from build123d import *

# Parameters (mm, degrees)
EXTRUDE_1_DEPTH     = 0.775
SKETCH_2_R          = 1.155
EXTRUDE_2_DEPTH     = 4.215
EXTRUDE_3_DEPTH     = 7.76
EXTRUDE_4_DEPTH     = 4.55
CUT_EXTRUDE_1_DEPTH = 2.5


with BuildPart() as part:
    # 스케치1 → 보스-돌출1 (new body, symmetric)
    with BuildSketch(Plane(origin=(0, 0, 0), x_dir=(0, 0, -1), z_dir=(1, 0, 0))):
        with BuildLine():
            Line((-2.73, 2.732106893), (-2.73, 2.198209499))
            ThreePointArc((-2.73, 2.198209499), (0, -3.505), (2.73, 2.198209499))
            Line((2.73, 2.198209499), (2.73, 2.732106893))
            ThreePointArc((2.73, 2.732106893), (0, 3.595), (-2.73, 2.732106893))
        make_face()
    extrude(amount=EXTRUDE_1_DEPTH, both=True)

    # 스케치2 → 보스-돌출2 (add, symmetric)
    with BuildSketch(Plane(origin=(0, 0, 0), x_dir=(0, 0, -1), z_dir=(1, 0, 0))):
        Circle(SKETCH_2_R)
    extrude(amount=EXTRUDE_2_DEPTH, both=True)

    # 스케치3 → 보스-돌출3 (add, symmetric)
    with BuildSketch(Plane(origin=(0, 0, 0), x_dir=(0, 0, -1), z_dir=(1, 0, 0))):
        with BuildLine():
            Line((-4.05, 2.73), (-2.73, 2.73))
            Line((-2.73, 2.73), (-2.73, 2.732106893))
            ThreePointArc((-2.73, 2.732106893), (0, 3.595), (2.73, 2.732106893))
            Line((2.73, 2.732106893), (2.73, 2.73))
            Line((2.73, 2.73), (4.05, 2.73))
            Line((4.05, 2.73), (4.05, 4.86))
            Line((4.05, 4.86), (-4.05, 4.86))
            Line((-4.05, 4.86), (-4.05, 2.73))
        make_face()
    extrude(amount=EXTRUDE_3_DEPTH, both=True)

    # 스케치4 → 보스-돌출4 (add)
    with BuildSketch(Plane(origin=(0, 4.86, 0), x_dir=(1, 0, 0), z_dir=(0, 1, 0))):
        with BuildLine():
            Line((-2.555, -2.44), (-5.335, -2.44))
            ThreePointArc((-5.335, -2.44), (-5.567190107, -1.747089472), (-6.17, -1.333982369))
            Line((-6.17, -1.333982369), (-6.17, 1.333982369))
            ThreePointArc((-6.17, 1.333982369), (-5.567190107, 1.747089472), (-5.335, 2.44))
            Line((-5.335, 2.44), (-2.555, 2.44))
            ThreePointArc((-2.555, 2.44), (-2.322809893, 1.747089472), (-1.72, 1.333982369))
            Line((-1.72, 1.333982369), (-1.72, -1.333982369))
            ThreePointArc((-1.72, -1.333982369), (-2.322809893, -1.747089472), (-2.555, -2.44))
        make_face()
    extrude_4 = extrude(amount=EXTRUDE_4_DEPTH)

    # 스케치5 → 컷-돌출1 (cut, symmetric)
    with BuildSketch(Plane.XY):
        Polygon((-6.17, 6.54), (-5.611088771, 9.41), (-6.17, 9.41), align=None)
    cut_extrude_1 = extrude(amount=CUT_EXTRUDE_1_DEPTH, both=True, mode=Mode.SUBTRACT)

    # 대칭 복사1: 보스-돌출4, 컷-돌출1 across plane
    add(extrude_4.mirror(Plane(origin=(0, 0, 0), x_dir=(0, 0, 1), z_dir=(1, 0, 0))))
    add(cut_extrude_1.mirror(Plane(origin=(0, 0, 0), x_dir=(0, 0, 1), z_dir=(1, 0, 0))), mode=Mode.SUBTRACT)


solid = part.part
Geometry: final body of the model. Coordinates: model frame, mm. A direction names the side the tool comes from. Round coordinates to 2 decimals unless told otherwise and drop trailing zeros. Loops run counter-clockwise (first coordinate to the right, second up) from the corner with the lowest first, then second, coordinate; pieces in that order, holes last. Notation, with made-up numbers: M -17.75,-22.75 L 39.25,-22.75 A10 ccw 39.25,-8.75 Z; hole C 31.25,17 d6. An arc over 180 degrees is marked long. One line per question, with ' | ' between items.
(1) Contact query for flat-ended pins moving along their axis: P1, Ø2, axis at y = 1, z = 0.5, coming from the +X side (3 decimals); P2, Ø0.7, axis at x = -3, z = 3.5, coming from the -Y side; P3, Ø1, axis at x = 3.5, y = 6.5, coming from the +Z side. Output: stop coordinate, or through.
Check result:
P1: stops at x = 4.215 | P2: stops at y = 2.73 | P3: stops at z = 2.44
(2) Cut plane C-C on z = 0. Return the cut outline in (x, y) (3 decimals).
Check result:
outline: M -7.76,3.595 L -0.775,3.595 L -0.775,1.155 L -4.215,1.155 L -4.215,-1.155 L -0.775,-1.155 L -0.775,-3.505 L 0.775,-3.505 L 0.775,-1.155 L 4.215,-1.155 L 4.215,1.155 L 0.775,1.155 L 0.775,3.595 L 7.76,3.595 L 7.76,4.86 L 6.17,4.86 L 6.17,6.54 L 5.611,9.41 L 1.72,9.41 L 1.72,4.86 L -1.72,4.86 L -1.72,9.41 L -5.611,9.41 L -6.17,6.54 L -6.17,4.86 L -7.76,4.86 Z
(3) Pull-direction query (X, two-part tool) for faces 6 (the flat face through (5.894, 7.955, 0.024)), 7 (the flat face through (0, 2.73, 3)), 8 (the cylindrical face through (2.33, 7.1, -1.76)); classes: +X half, -X half, draft (parallel to the pull), parting line (faces both ways), or undercut.
Check result:
face 6: +X half | face 7: draft | face 8: undercut
(4) Access query for faces 1 (the cylindrical face through (5.574, 7.103, -1.739)), 2 (the flat face through (1.72, 7, 0)), 3 (the flat face through (-4, 7, -2.44)), 4 (the cylindrical face through (2.52, 0.35, -1.1)), 5 (the flat face through (-4, 7, 2.44)). Directions: +Z, -Z, +X, -X, +Y, -Y. A direction counts if a zero-diameter tool reaches every point of the face in a straight line with its end or side. Return the directions, or none.
Check result:
face 1: -Z, +X, +Y | face 2: +Z, -Z, +Y | face 3: -Z, +X, -X, +Y | face 4: +X | face 5: +Z, +X, -X, +Y
(5) Material intervals for line 1 along X through (y, z) = (-1, -1.75) (3 decimals); line 2 along Y through (x, z) = (-6.5, 3); line 3 along X through (y, z) = (6.75, -1.75) (3 decimals), sorted ascending. Write a range as from..to.
Check result:
line 1: x = -0.775..0.775 | line 2: y = 2.73..4.86 | line 3: x = -5.565..-2.325, 2.325..5.565
(6) Cut plane B-B on y = 5.75. Return the cut outline in (x, z) (3 decimals).
Check result:
outline: M -6.17,-1.334 A1.15 cw -5.335,-2.44 L -2.555,-2.44 A1.15 cw -1.72,-1.334 L -1.72,1.334 A1.15 cw -2.555,2.44 L -5.335,2.44 A1.15 cw -6.17,1.334 Z; M 1.72,-1.334 A1.15 cw 2.555,-2.44 L 5.335,-2.44 A1.15 cw 6.17,-1.334 L 6.17,1.334 A1.15 cw 5.335,2.44 L 2.555,2.44 A1.15 cw 1.72,1.334 Z
(7) Cut plane D-D on y = 0. Return the cut outline in (x, z) (3 decimals), plus the area to 3 significant figures.
Check result:
outline: M -4.215,-1.155 L -0.775,-1.155 L -0.775,-3.505 L 0.775,-3.505 L 0.775,-1.155 L 4.215,-1.155 L 4.215,1.155 L 0.775,1.155 L 0.775,3.505 L -0.775,3.505 L -0.775,1.155 L -4.215,1.155 Z | area: 26.8 mm2
